Input: part model. Units: mm. Frame: model coordinates. A direction names the side the tool comes from. Coordinates: 2 decimals unless noted, no trailing zeros. Order: outer loops, then holes, each group sorted by start corner. A loop starts at its lowest first (then second) coordinate and runs counter-clockwise, first axis right, second up. Notation, with made-up numbers: (-32, 28.5) -> (25, 28.5) arc R19 ccw to (25, 48.5) -> close; hole circle Ø4 at (-0.75, 19.5). An arc over 180 degrees is marked (long way). One line per item, written item: value. Start each with the question number.
from build123d import *

# Parameters (mm, degrees)
F0_R     = 19.05
F1_DEPTH = 6.35
F2_T     = 0.762


with BuildPart() as f1:
    # F0 (on Top) → F1 (new body)
    with BuildSketch(Plane.XY):
        with BuildLine():
            Line((76.2, 57.15), (-120.4468, 57.15))
            ThreePointArc((-120.4468, 57.15), (-177.5968, 0), (-120.4468, -57.15))
            Line((-120.4468, -57.15), (76.2, -57.15))
            ThreePointArc((76.2, -57.15), (133.35, 0), (76.2, 57.15))
        make_face()
        with Locations((-44.2468, 0)):
            Circle(F0_R, mode=Mode.SUBTRACT)
        Circle(F0_R, mode=Mode.SUBTRACT)
    extrude(amount=F1_DEPTH)

    # F2
    f2_openings = [f1.faces().sort_by_distance(p)[0] for p in [
        (-22.1234, 0, 6.35),
    ]]
    offset(amount=F2_T, openings=f2_openings, kind=Kind.INTERSECTION)


solid = f1.part
1) Mould query, pull axis Y, two halves, no side actions, for faces 1 (the flat face through (-7.14, 17.02, 6.35)), 2 (the flat face through (-23, -57.912, 3)), 3 (the flat face through (-21, 57.912, 3)), 4 (the cylindrical face through (-15.12, -11.59, 3.13)). Classes: +Y half, -Y half, draft (parallel to the pull), parting line (faces both ways), or undercut.
2) Section query B-B, the plane y = 0. Return the cut outline in (x, z).
3) Section query D-D, the plane x = -87.5. Return the cut outline in (y, z).
4) Pin query (flat end, axial travel): pin 1 Ø3 at (x, z) = (86.5, 0.5) entering from -Y; pin 2 Ø2 at (y, z) = (-20, 2) entering from -X. Return the tip coordinate at first contact, or that it passes through.
5) Ray query, line 1 along Y through (x, z) = (0, 4.5); line 2 along Y through (x, z) = (-52.5, 1.25); line 3 along Y through (x, z) = (49.5, 1). Return the intervals inside material, ascending. Write a range as from..to.
6) Section query A-A, the plane z = 3.75. Return the cut outline in (x, y).
7) Access query for faces 5 (the cylindrical face through (-177.583, 1.257, 3.131)), 6 (the cylindrical face through (134.1, -1.27, 2.74)). Directions: +Z, -Z, +X, -X, +Y, -Y. A direction counts if a zero-diameter tool reaches every point of the face in a straight line with its end or side. Return the directions, or none.
8) Section query C-C, the plane x = 0. Return the cut outline in (y, z), plus the area to 3 significant figures.
Entries:
1. face 1: draft
1. face 2: -Y half
1. face 3: +Y half
1. face 4: undercut
2. outline: (-178.36, -0.76) -> (-62.53, -0.76) -> (-62.53, 6.35) -> (-63.3, 6.35) -> (-63.3, 0) -> (-177.6, 0) -> (-177.6, 6.35) -> (-178.36, 6.35) -> close; (-25.96, -0.76) -> (-18.29, -0.76) -> (-18.29, 6.35) -> (-19.05, 6.35) -> (-19.05, 0) -> (-25.2, 0) -> (-25.2, 6.35) -> (-25.96, 6.35) -> close; (18.29, -0.76) -> (134.11, -0.76) -> (134.11, 6.35) -> (133.35, 6.35) -> (133.35, 0) -> (19.05, 0) -> (19.05, 6.35) -> (18.29, 6.35) -> close
3. outline: (-57.91, -0.76) -> (57.91, -0.76) -> (57.91, 6.35) -> (57.15, 6.35) -> (57.15, 0) -> (-57.15, 0) -> (-57.15, 6.35) -> (-57.91, 6.35) -> close
4. pin 1: stops at y = -57.24
4. pin 2: stops at x = -175.15
5. line 1: y = -57.91..-57.15, -19.05..-18.29, 18.29..19.05, 57.15..57.91
5. line 2: y = -57.91..-57.15, -17.17..-16.32, 16.32..17.17, 57.15..57.91
5. line 3: y = -57.91..-57.15, 57.15..57.91
6. outline: (-120.45, -57.91) -> (76.2, -57.91) arc R57.91 ccw to (76.2, 57.91) -> (-120.45, 57.91) arc R57.91 ccw to start; circle Ø38.1 at (-44.25, 0); circle Ø38.1 at (0, 0); hole (-120.45, -57.15) -> (76.2, -57.15) arc R57.15 ccw to (76.2, 57.15) -> (-120.45, 57.15) arc R57.15 ccw to start; hole circle Ø36.58 at (-44.25, 0); hole circle Ø36.58 at (0, 0)
7. face 5: +Z
7. face 6: +Z, -Z, +X
8. outline: (-57.91, -0.76) -> (-18.29, -0.76) -> (-18.29, 6.35) -> (-19.05, 6.35) -> (-19.05, 0) -> (-57.15, 0) -> (-57.15, 6.35) -> (-57.91, 6.35) -> close; (18.29, -0.76) -> (57.91, -0.76) -> (57.91, 6.35) -> (57.15, 6.35) -> (57.15, 0) -> (19.05, 0) -> (19.05, 6.35) -> (18.29, 6.35) -> close
8. area: 79.7 mm2
